Part model, mm, in its own coordinate system. A direction names the side the tool comes from. Give positions to 0.01 mm unless a question says otherwise; leave off trailing zeros. Write each loop counter-clockwise with the first axis right and the second up, starting at its lowest first coordinate (ties: lowest second). Pieces come first, ordered by that corner, then holes.
```python
from build123d import *

# Parameters (mm, degrees)
SKETCH2_R           = 2
CUT_EXTRUDE1_DEPTH  = 10
BOSS_EXTRUDE1_DEPTH = 58
SKETCH4_R           = 10
BOSS_EXTRUDE2_DEPTH = 11


with BuildPart() as part:
    # Sketch1 → Revolve1 (revolve)
    with BuildSketch(Plane.XY, mode=Mode.PRIVATE) as revolve1_sk:
        Polygon((0, 4), (58, 4), (58, 30), (50, 30), (50, 8.5), (0, 8.5), align=None)
    revolve(revolve1_sk.sketch.rotate(Axis((0, 0, 0), (1, 0, 0)), 90), axis=Axis((0, 0, 0), (1, 0, 0)))

    # Sketch2 → Cut-Extrude1 (cut)
    with BuildSketch(Plane.ZY.offset(-50)):
        with Locations((0, 25)):
            Circle(SKETCH2_R)
        with Locations((17.67766953, 17.67766953)):
            Circle(SKETCH2_R)
        with Locations((25, 0)):
            Circle(SKETCH2_R)
        with Locations((17.67766953, -17.67766953)):
            Circle(SKETCH2_R)
        with Locations((0, -25)):
            Circle(SKETCH2_R)
        with Locations((-17.67766953, -17.67766953)):
            Circle(SKETCH2_R)
        with Locations((-25, 0)):
            Circle(SKETCH2_R)
        with Locations((-17.67766953, 17.67766953)):
            Circle(SKETCH2_R)
    extrude(amount=-CUT_EXTRUDE1_DEPTH, mode=Mode.SUBTRACT)

    # Sketch3 → Boss-Extrude1 (add, through all)
    with BuildSketch(Plane.ZY):
        with BuildLine():
            Line((-2.645751311, 3), (2.645751311, 3))
            ThreePointArc((2.645751311, 3), (0, 4), (-2.645751311, 3))
        make_face()
    extrude(amount=-BOSS_EXTRUDE1_DEPTH)

    # Sketch4 → Boss-Extrude2 (add)
    with BuildSketch(Plane.ZY.offset(-50)):
        with Locations(Location((0, 0, 0), (0, 0, 180))):
            Circle(SKETCH4_R)
        with BuildLine():
            Line((-2.645751311, 3), (2.645751311, 3))
            ThreePointArc((2.645751311, 3), (0, -4), (-2.645751311, 3))
        make_face(mode=Mode.SUBTRACT)
    extrude(amount=BOSS_EXTRUDE2_DEPTH)


solid = part.part
```
1) 3-axis set-ups, long thin cutter, end or side, ignore diameter. For faces 1 (the face through (45, 0, 10)), 2 (the face through (29, 3, 0)), 3 (the face through (58, 0, -6)): which of +Z, -Z, +X, -X, +Y, -Y reach the whole face in a straight line?
Answers follow:
face 1: -X
face 2: +X, -X
face 3: +Z, -Z, +X, +Y, -Y
2) Wall check: L1, parallel to Y at x = 52.75, z = 0; L2, parallel to X at y = -10, z = -21.5; L3, parallel to Y at x = 23, z = 0. Give the ranges that are in metal, low to high.
Answers follow:
L1: y = -30 to -27, -23 to -4, 3 to 23, 27 to 30
L2: x = 50 to 58
L3: y = -8.5 to -4, 3 to 8.5
3) Saw through at D-D, the plane x = 47.5. Write the cut outline in (y, z), then the cut area to 3 significant figures.
Answers follow:
outline: circle Ø20 at (0, 0); hole (3, -2.65) - (3, 2.65) arc R4 ccw (long way) to start
area: 268 mm2
4) Pin check, flat tips, straight feed: pin 1 Ø4 at (x, z) = (35, 9.5) entering from +Y; pin 2 Ø3 at (x, z) = (21, -6) entering from +Y; pin 3 Ø6.5 at (y, z) = (-17.68, -17.68) entering from -X. Stop position of each tip, or through.
Answers follow:
pin 1: stops at y = 4
pin 2: stops at y = 7.21
pin 3: stops at x = 50
5) Saw through at A-A, the plane y = 0. Write the cut outline in (x, z), then the cut area to 3 significant figures.
Answers follow:
outline: (0, -8.5) - (39, -8.5) - (39, -10) - (50, -10) - (50, -23) - (58, -23) - (58, -4) - (0, -4) - close; (0, 4) - (58, 4) - (58, 23) - (50, 23) - (50, 10) - (39, 10) - (39, 8.5) - (0, 8.5) - close; (50, -30) - (58, -30) - (58, -27) - (50, -27) - close; (50, 27) - (58, 27) - (58, 30) - (50, 30) - close
area: 835 mm2
6) Two-plate mould, pull along Y, no slides. Class faces 4 (the face through (29, -4, 0)), 5 (the face through (0, 4, 0)), 6 (the face through (53.944, 19.029, 16.204)), 7 (the face through (53.944, -25.296, 16.128)): +Y half, -Y half, draft (parallel to the pull), parting line (faces both ways), or undercut.
Answers follow:
face 4: undercut
face 5: draft
face 6: undercut
face 7: parting line
7) Saw through at C-C, the plane y = 25. Write the cut outline in (x, z).
Answers follow:
outline: (50, -16.58) - (58, -16.58) - (58, -2) - (50, -2) - close; (50, 2) - (58, 2) - (58, 16.58) - (50, 16.58) - close
8) Saw through at B-B, the plane z = 18. Write the cut outline in (x, y), then the cut area to 3 significant figures.
Answers follow:
outline: (50, -24) - (58, -24) - (58, -19.65) - (50, -19.65) - close; (50, -15.7) - (58, -15.7) - (58, 15.7) - (50, 15.7) - close; (50, 19.65) - (58, 19.65) - (58, 24) - (50, 24) - close
area: 321 mm2
